Could you check a few things on this drawing? It's one solid part, dimensions in mm from its lowest x, y, z. Round coordinates to 2 decimals unless told otherwise and drop trailing zeros. Loops run counter-clockwise (first coordinate to the right, second up) from the corner with the lowest first, then second, coordinate; pieces in that order, holes last. Notation, with made-up numbers: M 36,61.25 L 52,61.25 A30 cw 52,97.25 Z; hole C 65,63 d8. An arc over 180 degrees is marked long. Use a Markdown table: item, result. Add a question column.
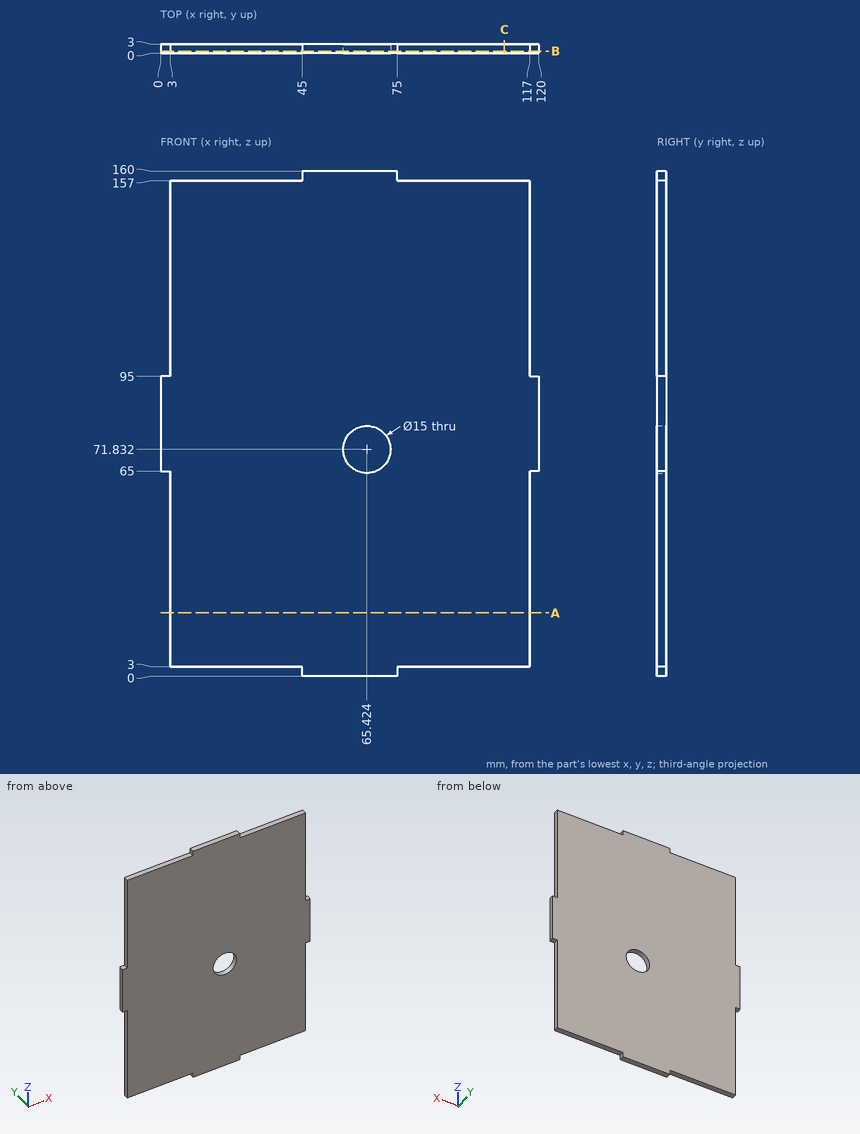
(1) Suppose I cut it at A-A on z = 20. List the corners of the cut face in (x, y) for me, and give its area (3 significant figures).
(2) If I drill on probe 1 along Z at (x, y) = (7.5, 0.4); probe 2 along X at (y, z) = (0.65, 35); probe 3 along X at (y, z) = (1.15, 76), over which ranges is the centre line in solid material (lowest first)? Write a range as [from, to].
(3) Suppose I cut it at C-C on x = 109. List the corners of the cut face in (y, z) for me.
(4) I'm going to push flat-ended pins straight in: pin 1 (1 mm diameter, centred on y = 2, z = 125.5, fed in from +X); pin 2 (10 mm diameter, centred on x = 55, z = 110.5, fed in from -Y); pin 3 (1.5 mm diameter, centred on x = 2, y = 2, fed in from +Z); pin 4 (1.5 mm diameter, centred on x = 18.5, y = 1.5, fed in from -Z). Where does each tip first touch, or does it pass through?
(5) Suppose I cut it at B-B on y = 0.75. List the corners of the cut face in (x, z) for me, and give its area (3 significant figures).
Results below:
| question | item | result |
|---|---|---|
| 1 | outline | M 3,0 L 117,0 L 117,3 L 3,3 Z |
| 1 | area | 342 mm² |
| 2 | probe 1 | z = [3, 157] |
| 2 | probe 2 | x = [3, 117] |
| 2 | probe 3 | x = [0, 59.19], [71.66, 120] |
| 3 | outline | M 0,3 L 3,3 L 3,157 L 0,157 Z |
| 4 | pin 1 | stops at x = 117 |
| 4 | pin 2 | stops at y = 0 |
| 4 | pin 3 | stops at z = 95 |
| 4 | pin 4 | stops at z = 3 |
| 5 | outline | M 0,65 L 3,65 L 3,3 L 45,3 L 45,0 L 75,0 L 75,3 L 117,3 L 117,65 L 120,65 L 120,95 L 117,95 L 117,157 L 75,157 L 75,160 L 45,160 L 45,157 L 3,157 L 3,95 L 0,95 Z; hole C 65.42,71.83 d15 |
| 5 | area | 17,700 mm² |
